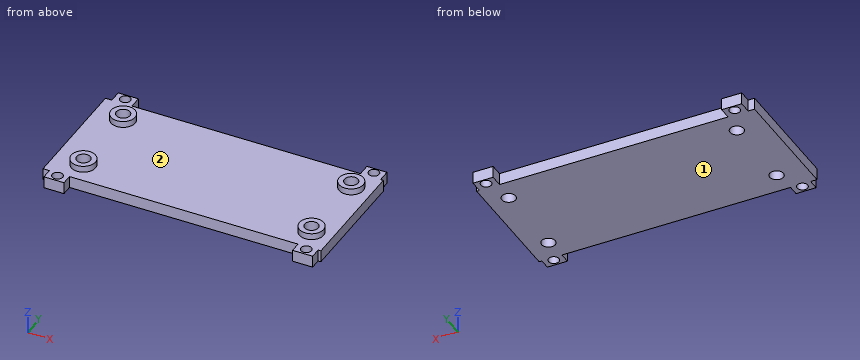
from build123d import *

# Parameters (mm, degrees)
PROFILE_R         = 1.15
PROFILE_R_2       = 1.5
EXTRUDE_266_DEPTH = 2.6
EXTRUDE_START     = 2.6
PROFILE_2_R       = 2.65
PROFILE_2_R_2     = 1.5
EXTRUDE_339_DEPTH = 1.4


with BuildPart() as part:
    # profile → Extrude 266 (new body)
    with BuildSketch(Plane.XY):
        Polygon((-43.1, 4), (-41.7, 4), (-41.7, 1.65), (-37.3, 1.65), (-37.3, 4), (12.8, 4), (12.8, 1.65), (17.2, 1.65), (17.2, 4), (17.8, 4), (17.8, 30.75), (17.2, 30.75), (17.2, 33.5), (12.8, 33.5), (12.8, 30.75), (-37.3, 30.75), (-37.3, 33.5), (-41.7, 33.5), (-41.7, 30.75), (-43.1, 30.75), align=None)
        with Locations((-39.5, 3.2)):
            Circle(PROFILE_R, mode=Mode.SUBTRACT)
        with Locations((15, 3.2)):
            Circle(PROFILE_R, mode=Mode.SUBTRACT)
        with Locations((-39.5, 32.2)):
            Circle(PROFILE_R, mode=Mode.SUBTRACT)
        with Locations((15, 32.2)):
            Circle(PROFILE_R, mode=Mode.SUBTRACT)
        with Locations((-36.75, 8.9)):
            Circle(PROFILE_R_2, mode=Mode.SUBTRACT)
        with Locations((13.25, 8.9)):
            Circle(PROFILE_R_2, mode=Mode.SUBTRACT)
        with Locations((-36.75, 25.9)):
            Circle(PROFILE_R_2, mode=Mode.SUBTRACT)
        with Locations((13.25, 25.9)):
            Circle(PROFILE_R_2, mode=Mode.SUBTRACT)
    extrude(amount=EXTRUDE_266_DEPTH)

    # profile 2 → Extrude 339 (add)
    # profile 1 of 4: a face of its own
    with BuildSketch(Plane.XY.offset(EXTRUDE_START)):
        with Locations((-36.75, 8.9)):
            Circle(PROFILE_2_R)
        with Locations((-36.75, 8.9)):
            Circle(PROFILE_2_R_2, mode=Mode.SUBTRACT)
    # profile 2 of 4: a face of its own
    with BuildSketch(Plane.XY.offset(EXTRUDE_START)):
        with Locations((13.25, 8.9)):
            Circle(PROFILE_2_R)
        with Locations((13.25, 8.9)):
            Circle(PROFILE_2_R_2, mode=Mode.SUBTRACT)
    # profile 3 of 4: a face of its own
    with BuildSketch(Plane.XY.offset(EXTRUDE_START)):
        with Locations((-36.75, 25.9)):
            Circle(PROFILE_2_R)
        with Locations((-36.75, 25.9)):
            Circle(PROFILE_2_R_2, mode=Mode.SUBTRACT)
    # profile 4 of 4: a face of its own
    with BuildSketch(Plane.XY.offset(EXTRUDE_START)):
        with Locations((13.25, 25.9)):
            Circle(PROFILE_2_R)
        with Locations((13.25, 25.9)):
            Circle(PROFILE_2_R_2, mode=Mode.SUBTRACT)
    extrude(amount=EXTRUDE_339_DEPTH)


solid = part.part
Can you work these out from the model? Positions are in its coordinate system, mm. Face numbers are marked on the shaded views. Coordinates: 2 decimals unless noted, no trailing zeros. Order: outer loops, then holes, each group sorted by start corner. A loop starts at its lowest first (then second) coordinate and runs counter-clockwise, first axis right, second up. Notation, with made-up numbers: M 76.25,82 L 87.25,82 A11 ccw 87.25,93 Z; hole C -29,66 d7. An arc over 180 degrees is marked long. Write item = value, one per line.
(1) I need wall thicknesses on line 1 along Y through (x, z) = (13.25, 1); line 2 along Y through (x, z) = (15, 1.1); line 3 along Y through (x, z) = (-8, 1.45). Which ranges of each line are inside material? Lowest first, please. Write a range as [from, to].
Results are:
line_1 = [1.65, 7.4], [10.4, 24.4], [27.4, 33.5]
line_2 = [1.65, 2.05], [4.35, 31.05], [33.35, 33.5]
line_3 = [4, 30.75]
(2) For pin 1 Ø9.5 at (x, y) = (-19, 15) entering from +Z; pin 2 Ø1.5 at (x, z) = (-42.5, 1) entering from +Y; pin 3 Ø10 at (x, y) = (-21, 10) entering from -Z; pin 4 Ø1.3 at (x, z) = (-14.5, 1.5) entering from -Y, each with a flat end and sliding along its axis, tell me the tip position at first contact or that it passes through.
Results are:
pin_1 = 2.6
pin_2 = 30.75
pin_3 = 0
pin_4 = 4
(3) Suppose I cut it at C-C on x = -36. Please give me the cut outline in (y, z), plus the area to 3 significant figures.
Results are:
outline = M 4,0 L 7.6,0 L 7.6,4 L 6.36,4 L 6.36,2.6 L 4,2.6 Z; M 10.2,0 L 24.6,0 L 24.6,4 L 23.36,4 L 23.36,2.6 L 11.44,2.6 L 11.44,4 L 10.2,4 Z; M 27.2,0 L 30.75,0 L 30.75,2.6 L 28.44,2.6 L 28.44,4 L 27.2,4 Z
area = 63.0 mm2
(4) If we mould it in two halves opening along X, with no side actions, what happens to the marked faces 1 and 2? For each: pulls with the +X half, pulls with the -X half, needs draft (parallel to the pull), parting line crosses it, or undercut.
Results are:
face_1 = needs draft
face_2 = undercut
(5) Suppose I cut it at A-A on y = 3.2. Please give me the cut outline in (x, z).
Results are:
outline = M -41.7,0 L -40.65,0 L -40.65,2.6 L -41.7,2.6 Z; M -38.35,0 L -37.3,0 L -37.3,2.6 L -38.35,2.6 Z; M 12.8,0 L 13.85,0 L 13.85,2.6 L 12.8,2.6 Z; M 16.15,0 L 17.2,0 L 17.2,2.6 L 16.15,2.6 Z
(6) Suppose I cut it at D-D on y = 13. Please give me the cut outline in (x, z).
Results are:
outline = M -43.1,0 L 17.8,0 L 17.8,2.6 L -43.1,2.6 Z
(7) Suppose I cut it at B-B on y = 8.9. Please give me the cut outline in (x, z), plus the area to 3 significant figures.
Results are:
outline = M -43.1,0 L -38.25,0 L -38.25,4 L -39.4,4 L -39.4,2.6 L -43.1,2.6 Z; M -35.25,0 L 11.75,0 L 11.75,4 L 10.6,4 L 10.6,2.6 L -34.1,2.6 L -34.1,4 L -35.25,4 Z; M 14.75,0 L 17.8,0 L 17.8,2.6 L 15.9,2.6 L 15.9,4 L 14.75,4 Z
area = 149 mm2
